Geometry: see drawing. Coordinates: mm, zero at the bounding-box minimum. A direction names the side the tool comes from. Round coordinates to 2 decimals unless told otherwise and drop trailing zeros. Loops run counter-clockwise (first coordinate to the right, second up) from the corner with the lowest first, then second, coordinate; pieces in that order, holes last. Notation, with made-up numbers: (1, 81) - (25, 81) arc R8 ccw to (25, 94) - close; hole circle Ø9 at (45.25, -28). An arc over 180 degrees is marked (long way). Return JSON: item names as keys, results as strings. Group by question number.
1. Section A-A on x = 7.25. Return loops of the section in (y, z).
2. First-contact query: pin 1 Ø5 at (x, z) = (1.5, 26.5) entering from -Y; pin 2 Ø4 at (x, y) = (5.05, 4.38) entering from -Z; pin 3 Ø2 at (x, z) = (6, 14.5) entering from +Y (3 decimals). Flat tips, straight axial feed; report the tip coordinate or a pass-through.
3. Draft query along X for the marked faces 1, 2 and 3. Return one class per face: +X half, -X half, draft (parallel to the pull), parting line (faces both ways), or undercut.
4. Section B-B on y = 3.5. Return loops of the section in (x, z) (1 decimal).
5. Section C-C on z = 16. Return loops of the section in (x, y) (1 decimal).
6. Material intervals for probe 1 along Z at (x, y) = (1, 3.75); probe 2 along X at (y, z) = (5.75, 4) (1 decimal); probe 3 along X at (y, z) = (6, 26), sorted ascending.
7. Section D-D on y = 8.25. Return loops of the section in (x, z).
8. Set-up query: the marked faces 4 and 5. Return all of +Z, -Z, +X, -X, +Y, -Y with unobstructed straight access to the full face (end or side cutting, diameter ignored); none if empty.
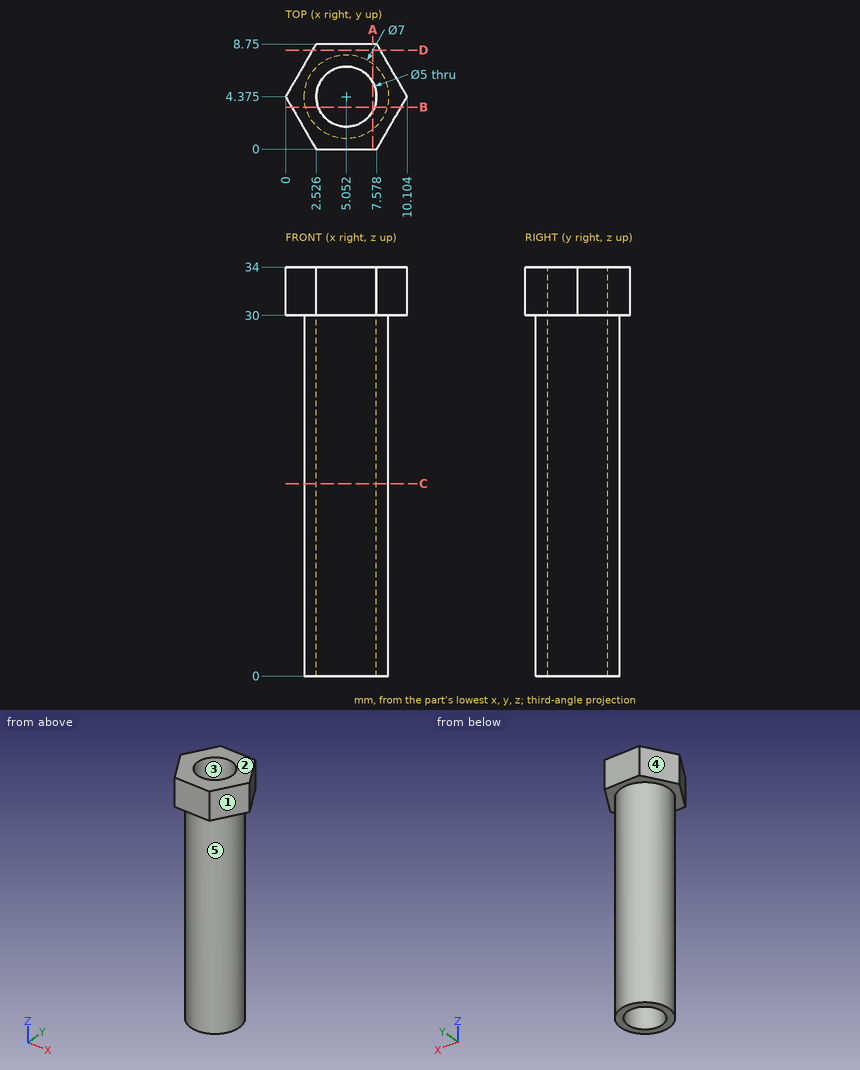
Taken from the geometry:
{
 "1": {"outline": "(0, 30) - (1.65, 30) - (1.65, 0) - (3.18, 0) - (3.18, 34) - (0, 34) - close; (5.57, 0) - (7.1, 0) - (7.1, 30) - (8.75, 30) - (8.75, 34) - (5.57, 34) - close"},
 "2": {"pin 1": "y = 1.04", "pin 2": "through", "pin 3": "y = 7.875"},
 "3": {"face 1": "+X half", "face 2": "draft", "face 3": "undercut"},
 "4": {"outline": "(0.5, 30) - (1.7, 30) - (1.7, 0) - (2.7, 0) - (2.7, 34) - (0.5, 34) - close; (7.4, 0) - (8.4, 0) - (8.4, 30) - (9.6, 30) - (9.6, 34) - (7.4, 34) - close"},
 "5": {"outline": "circle Ø7 at (5.1, 4.4); hole circle Ø5 at (5.1, 4.4)"},
 "6": {"probe 1": "30 to 34", "probe 2": "1.8 to 3, 7.1 to 8.3", "probe 3": "1.95 to 3.15, 6.95 to 8.15"},
 "7": {"outline": "(2.24, 30) - (7.87, 30) - (7.87, 34) - (2.24, 34) - close"},
 "8": {"face 4": "+Z, -Z, -X, +Y", "face 5": "-Z"}
}
